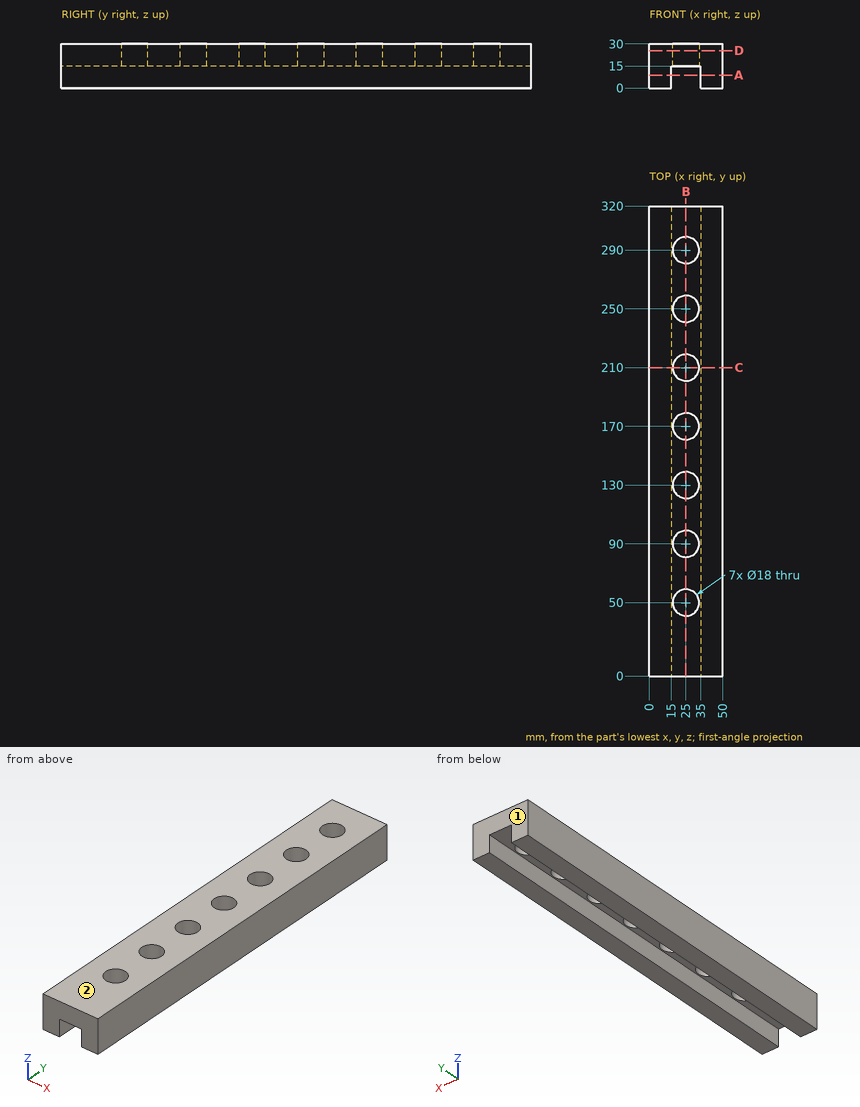
Could you check a few things on this drawing? It's one solid part, dimensions in mm from its lowest x, y, z. Give positions to 0.01 mm unless a question says otherwise; leave off trailing zeros. Order: outer loops, then holes, each group sorted by start corner. A loop starts at its lowest first (then second) coordinate and runs counter-clockwise, first axis right, second up. Notation, with made-up numbers: (66.5, 61.25) -> (72.5, 61.25) arc R21 cw to (72.5, 82.25) -> close; hole circle Ø2 at (67.5, 87.5). An arc over 180 degrees is marked (long way). Answer in a Markdown table with one row per item. Add a question column.
Item 1: Please list where these lines run through material, in increasing order: probe 1 along X at (y, z) = (129.5, 11.25); probe 2 along X at (y, z) = (202.5, 16.25); probe 3 along Z at (x, y) = (32.5, 216.5).
Item 2: Imagine slicing it at D-D (z = 25.5). List the corners of the cut face in (x, y) for me, and give its area (3 significant figures).
Item 3: We'd pull the mould along Z, two halves only. Please class the marked faces 1 and 2: pulls with the +Z half, pulls with the -Z half, needs draft (parallel to the pull), parting line crosses it, or undercut.
Item 4: Imagine slicing it at A-A (z = 8.75). List the corners of the cut face in (x, y) for me.
Item 5: Imagine slicing it at C-C (y = 210). List the corners of the cut face in (x, z) for me, and give its area (3 significant figures).
Item 6: I'm going to push flat-ended pins straight in: P1, Ø6, axis at x = 25.5, y = 234.5, coming from the -Z side; P2, Ø11, axis at x = 25, y = 90, coming from the -Z side. Where does each tip first touch, or does it pass through?
Item 7: Imagine slicing it at B-B (x = 25). Count the separate pieces of the cut face and the enclosed holes in it, and give its area (3 significant figures).
Result:
| question | item | result |
|---|---|---|
| 1 | probe 1 | 0 to 15, 35 to 50 |
| 1 | probe 2 | 0 to 20.03, 29.97 to 50 |
| 1 | probe 3 | 15 to 30 |
| 2 | outline | (0, 0) -> (50, 0) -> (50, 320) -> (0, 320) -> close; hole circle Ø18 at (25, 50); hole circle Ø18 at (25, 90); hole circle Ø18 at (25, 130); hole circle Ø18 at (25, 170); hole circle Ø18 at (25, 210); hole circle Ø18 at (25, 250); hole circle Ø18 at (25, 290) |
| 2 | area | 14,200 mm2 |
| 3 | face 1 | needs draft |
| 3 | face 2 | pulls with the +Z half |
| 4 | outline | (0, 0) -> (15, 0) -> (15, 320) -> (0, 320) -> close; (35, 0) -> (50, 0) -> (50, 320) -> (35, 320) -> close |
| 5 | outline | (0, 0) -> (15, 0) -> (15, 15) -> (16, 15) -> (16, 30) -> (0, 30) -> close; (34, 15) -> (35, 15) -> (35, 0) -> (50, 0) -> (50, 30) -> (34, 30) -> close |
| 5 | area | 930 mm2 |
| 6 | P1 | z = 15 |
| 6 | P2 | through |
| 7 | separate pieces | 8 |
| 7 | enclosed holes | 0 |
| 7 | area | 2,910 mm2 |
